For this review, take the finished solid that the model builds, in its own axes (mm). A direction names the side the tool comes from. Coordinates: 2 decimals unless noted, no trailing zeros. Write each loop counter-clockwise with the first axis right and the second up, starting at its lowest first coordinate (ties: lowest second). Pieces come first, ordered by that corner, then holes. Notation, with made-up numbers: (67.25, 86.25) - (103.25, 86.25) arc R15 ccw to (103.25, 91.25) - close; hole circle Ø3 at (-18.75, 27). An arc over 180 degrees is marked (long way). Write each question's results on one line, items separated by ' | '.
Autodesk Inventor part; units mm, degrees
ref_plane "YZ Plane" through (0, 0, 0) normal (1, 0, 0) x (0, 1, 0)
ref_plane "XZ Plane" through (0, 0, 0) normal (0, 1, 0) x (-1, 0, 0)
ref_plane "XY Plane" through (0, 0, 0) normal (0, 0, 1) x (1, 0, 0)
sketch "スケッチ1" plane through (0, 0, 0) normal (0, 0, 1) x (1, 0, 0)
  line L0 (0, 0) -> (45, 0)
  line L1 (45, 0) -> (45, 1.5)
  line L2 (45, 1.5) -> (0, 1.5)
  line L3 (0, 1.5) -> (0, 0)
  line L4 (0, 0) -> (0, 2.75)
  line L5 (0, 0) -> (-2, 0)
  line L6 (-2, 0) -> (0, 0)
  line L7 (-2, 0) -> (-2, 1.15)
  line L8 (0, 0) -> (-2, 0)
  line L9 (-2, 0) -> (-2, 2.75)
  line L10 (-2, 2.75) -> (0, 2.75)
  line L11 (0, 2.75) -> (0, 0)
  dimension "d0" = 1.5
  dimension "d1" = 45
  dimension "d3" = 2
  dimension "d4" = 2.75
  dimension "d5" = 1.15
revolve "回転1" add sketch "スケッチ1" angle 360 about axis through (-2, 0, 0) along (1, 0, 0)
sketch "スケッチ2" plane through (-2, 0, 0) normal (-1, 0, 0) x (0, 0, 1)
  line L0 (-0.575, 0.9959) -> (0.575, 0.9959)
  line L1 (0.575, 0.9959) -> (1.15, 0)
  line L2 (1.15, 0) -> (0.575, -0.9959)
  line L3 (0.575, -0.9959) -> (-0.575, -0.9959)
  line L4 (-0.575, -0.9959) -> (-1.15, 0)
  line L5 (-1.15, 0) -> (-0.575, 0.9959)
  point P0 (0, 0)
  point P1 (0, 0)
  point P2 (0, 0)
  dimension "d10" = 1.15
  dimension "d11" = 1.9919
extrude "押し出し1" cut sketch "スケッチ2" against normal blind 1.4
fillet "フィレット1" radius 0.2 6 edges at (-0.6, 0.9959, 0) (-0.6, 0.498, 0.8625) (-0.6, 0.498, -0.8625) (-0.6, -0.498, -0.8625) (-0.6, -0.9959, 0) (-0.6, -0.498, 0.8625)
fillet "フィレット2" radius 0.1 1 edges at (0, -1.5, 0)
fillet "フィレット3" radius 0.1 1 edges at (45, -1.5, 0)
thread "ねじ2"
properties part number "ネジキャップM3L45" material "鋼"
Q1. For pin 1 (2 mm diameter, centred on x = 29, y = -2, fed in from +Z); pin 2 (1 mm diameter, centred on x = 16.5, y = 0, fed in from +Z), all flat-tipped, find the tip position at first contact; note any pin that passes through.
Results found:
pin 1: z = 1.12 | pin 2: z = 1.5
Q2. For faces 4 (the face through (0, 2, 0)), 5 (the face through (-2, 1.2, 0)), 6 (the face through (-1.408, -0.491, 0.867)), list the 3-axis set-ups (+Z, -Z, +X, -X, +Y, -Y) from which the entire face can be reached by the end or side of a thin tool; tool diameter is ignored.
Results found:
face 4: +X | face 5: +Z, -Z, -X, +Y, -Y | face 6: -X
Q3. Take a section at A-A on z = 0. State the section outline as (x, y) points, plus the area to 3 significant figures.
Results found:
outline: (-2, -2.75) - (0, -2.75) - (0, -1.6) arc R0.1 cw to (0.1, -1.5) - (44.9, -1.5) arc R0.1 ccw to (45, -1.4) - (45, 1.4) arc R0.1 ccw to (44.9, 1.5) - (0.1, 1.5) arc R0.1 cw to (0, 1.6) - (0, 2.75) - (-2, 2.75) - (-2, 1) - (-0.8, 1) arc R0.2 cw to (-0.6, 0.8) - (-0.6, -0.8) arc R0.2 cw to (-0.8, -1) - (-2, -1) - close | area: 143 mm2
Q4. Take a section at B-B on x = 19. State the section outline as (y, z) points.
Results found:
outline: circle Ø3 at (0, 0)
Q5. Mouldability with a two-part tool opening along Y and no side actions: class faces 1 (the face through (45, 0, 0)), 2 (the face through (-0.6, 0, 0)), 3 (the face through (-0.986, -0.596, -2.685)) as pulls with the +Y half, pulls with the -Y half, needs draft (parallel to the pull), parting line crosses it, or undercut.
Results found:
face 1: needs draft | face 2: undercut | face 3: parting line crosses it
Q6. Wall thickness on line 1 along Z through (x, y) = (24, 0); line 2 along X through (y, z) = (1.2, 2.15); line 3 along Y through (x, z) = (6.5, 0.55): over which ranges is each line inside the solid? List them lowest first. Write a range as from..to.
Results found:
line 1: -1.5..1.5 | line 2: -2..0 | line 3: -1.4..1.4
Q7. Take a section at C-C on y = -2.2. State the section outline as (x, z) points, plus the area to 3 significant figures.
Results found:
outline: (-2, -1.65) - (0, -1.65) - (0, 1.65) - (-2, 1.65) - close | area: 6.60 mm2
